from build123d import *

# Parameters (mm, degrees)
SKETCH2_R           = 2.5
BOSS_EXTRUDE1_DEPTH = 45
BOSS_EXTRUDE2_DEPTH = 5


with BuildPart() as part:
    # Sweep1: sweep along a curve in space
    with BuildLine() as sweep1_path:
        Line((-40, -30.35817133, -2.7), (-40, -114.302855497, -45))
        ThreePointArc((-34, -25, 0), (-38.242640687, -26.569372048, -0.790811691), (-40, -30.35817133, -2.7))
        Line((-6, -25, 0), (-34, -25, 0))
        ThreePointArc((-6, -25, 0), (-1.757359313, -23.242640687, 0), (0, -19, 0))
        Line((0, -6, 0), (0, -19, 0))
        ThreePointArc((-6, 0, 0), (-1.757359313, -1.757359313, 0), (0, -6, 0))
        Line((-6, 0, 0), (-19, 0, 0))
    # Sketch2 → Sweep1 (sweep)
    with BuildSketch(Plane(origin=(-19, 0, 0), x_dir=(0, 0, -1), z_dir=(1, 0, 0))):
        Circle(SKETCH2_R)
    sweep(path=sweep1_path.line)

    # Sketch3 → Boss-Extrude1 (add)
    with BuildSketch(Plane(origin=(0, -109.240355497, -55.046571243), x_dir=(1, 0, 0), z_dir=(0, -0.8930285549745877, -0.45000000000000007))):
        with BuildLine():
            Line((-37.5, 11.25), (-37.5, 12.5))
            ThreePointArc((-37.5, 12.5), (-40, 15), (-42.5, 12.5))
            Line((-42.5, 12.5), (-42.5, 11.25))
            ThreePointArc((-42.5, 11.25), (-40, 13.75), (-37.5, 11.25))
        make_face()
        with BuildLine():
            ThreePointArc((-42.5, 11.25), (-40, 8.75), (-37.5, 11.25))
            ThreePointArc((-37.5, 11.25), (-40, 13.75), (-42.5, 11.25))
        make_face()
        with BuildLine():
            Line((-37.5, 10), (-37.5, 11.25))
            ThreePointArc((-37.5, 11.25), (-40, 8.75), (-42.5, 11.25))
            Line((-42.5, 11.25), (-42.5, 10))
            ThreePointArc((-42.5, 10), (-40, 7.5), (-37.5, 10))
        make_face()
    extrude(amount=-BOSS_EXTRUDE1_DEPTH)

    # Sketch4 → Boss-Extrude2 (add)
    with BuildSketch(Plane.ZY.offset(42.5)):
        Polygon((-39.833714306, -106.828098503), (-29.963286264, -108.432670178), (-33.083714306, -93.432670178), align=None)
    extrude(amount=-BOSS_EXTRUDE2_DEPTH)


solid = part.part
Work out the finished part from the listing and answer in its coordinate system (mm). A direction names the side the tool comes from. Round coordinates to 2 decimals unless told otherwise and drop trailing zeros. Write each loop counter-clockwise with the first axis right and the second up, starting at its lowest first coordinate (ties: lowest second). Pieces come first, ordered by that corner, then holes. Notation, with made-up numbers: (42.25, -20.5) - (84.25, -20.5) arc R18 ccw to (84.25, 3.5) - close; hole circle Ø1 at (83, 44). An arc over 180 degrees is marked (long way). Answer in a Markdown table with one row per item. Add a question column.
1. Given pin 1 (4 mm diameter, centred on y = -75.5, z = -20, fed in from +X); pin 2 (6.5 mm diameter, centred on y = -86.5, z = -31.5, fed in from +X); pin 3 (6 mm diameter, centred on x = -17, z = -5, fed in from +Y), each flat-ended and moving along its own axis, determine where each tip first touches the part or whether it passes through.
2. Find the intervals of material crossed by line 1 along Y through (x, z) = (-6.5, -1.5); line 2 along Z through (x, y) = (-39, -54.5); line 3 along X through (y, z) = (-73.5, -25.5), in increasing order. Write a range as from..to.
3. The mould has two halves that part along Y. Classify faces 1 (the flat face through (-40.035, -107.797, -33.871)), 2 (the cylindrical face through (-40.055, -92.804, -38.365)), 3 (the cylindrical face through (-12.41, -2.44, 0.54)): +Y half, -Y half, draft (parallel to the pull), parting line (faces both ways), or undercut.
4. A cutting plane is placed at A-A, the plane x = -7.5. Determine the outline of the cut face in (y, z), and give its area (3 significant figures).
5. For faces 4 (the cylindrical face through (-20.2, -27.48, 0.33)), 5 (the cylindrical face through (-39.95, -111.68, -39.48)), 6 (the flat face through (-39.83, -72.9, -27.16)), 7 (the flat face through (-39.83, -75.34, -22.32)), determine the directions among +Z, -Z, +X, -X, +Y, -Y from which every point of the face is accessible in a straight line to the end or side of a thin tool.
6. A cutting plane is placed at B-B, the plane x = -32. Determine the outline of the cut face in (y, z), and give its area (3 significant figures).
Worked out:
| question | item | result |
|---|---|---|
| 1 | pin 1 | x = -38.3 |
| 1 | pin 2 | x = -37.5 |
| 1 | pin 3 | y = 1.5 |
| 2 | line 1 | -27..-23, -2..2 |
| 2 | line 2 | -17.43..-12.3 |
| 2 | line 3 | -42.31..-37.69 |
| 3 | face 1 | -Y half |
| 3 | face 2 | +Y half |
| 3 | face 3 | undercut |
| 4 | outline | circle Ø5 at (-25, 0); circle Ø5 at (0, 0) |
| 4 | area | 39.3 mm^2 |
| 5 | face 4 | none |
| 5 | face 5 | -Y |
| 5 | face 6 | +Y |
| 5 | face 7 | +Z |
| 6 | outline | circle Ø5 at (-25, 0) |
| 6 | area | 19.6 mm^2 |
